from build123d import *

# Parameters (mm, degrees)
SKETCH1_W           = 80
SKETCH1_H           = 198
BOSS_EXTRUDE1_DEPTH = 5
SKETCH2_R           = 3.75
BOSS_EXTRUDE2_DEPTH = 7.5
CUT_EXTRUDE1_DEPTH  = 88.5
FILLET2_R           = 2
CUT_EXTRUDE2_START  = -5
SKETCH4_R           = 3
CUT_EXTRUDE2_DEPTH  = 2


with BuildPart() as part:
    # Sketch1 → Boss-Extrude1 (new body)
    with BuildSketch(Plane(origin=(0, 0, 0), x_dir=(1, 0, 0), z_dir=(0, 1, 0))):
        Rectangle(SKETCH1_W, SKETCH1_H)
    extrude(amount=BOSS_EXTRUDE1_DEPTH)

    # Sketch2 → Boss-Extrude2 (add)
    with BuildSketch(Plane.ZY.offset(40)):
        with Locations((-64.928905814, 3.75)):
            Circle(SKETCH2_R)
        with Locations((59.5, 3.75)):
            Circle(SKETCH2_R)
    boss_extrude2 = extrude(amount=BOSS_EXTRUDE2_DEPTH)

    # Mirror1: Boss-Extrude2 across plane
    add(boss_extrude2.mirror(Plane(origin=(0, 0, 0), x_dir=(0, 0, 1), z_dir=(1, 0, 0))))

    # Sketch3 → Cut-Extrude1 (cut, through all)
    with BuildSketch(Plane.ZY.offset(40)):
        Polygon((-99, 5), (-72.932513489, -1.759148434), (-103.799311702, -1.759148434), align=None)
    extrude(amount=-CUT_EXTRUDE1_DEPTH, mode=Mode.SUBTRACT)

    # Fillet2
    fillet2_edges = [part.edges().sort_by_distance(p)[0] for p in [
        (40, 2.5, -89.358442796),
        (-40, 2.5, -89.358442796),
    ]]
    fillet(fillet2_edges, radius=FILLET2_R)

    # Sketch4 → Cut-Extrude2 (cut)
    with BuildSketch(Plane.XZ.offset(CUT_EXTRUDE2_START)):
        with Locations((-35, -69.716885591)):
            Circle(SKETCH4_R)
        with Locations((35, -69.716885591)):
            Circle(SKETCH4_R)
        with Locations((-35, 94)):
            Circle(SKETCH4_R)
        with Locations((35, 94)):
            Circle(SKETCH4_R)
    extrude(amount=CUT_EXTRUDE2_DEPTH, mode=Mode.SUBTRACT)


solid = part.part
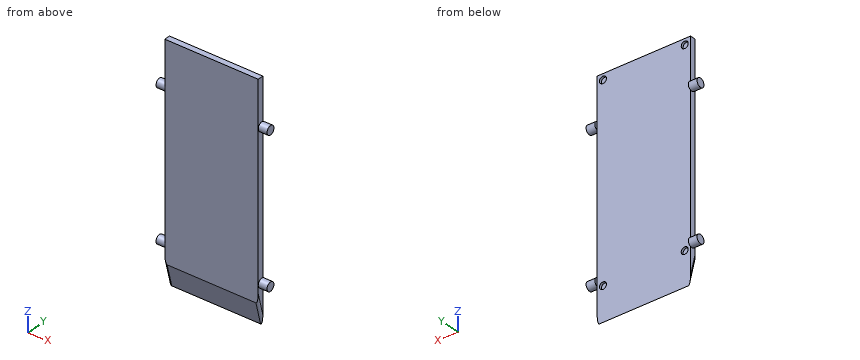
Work out the finished part from the listing and answer in its coordinate system (mm). Coordinates: 2 decimals unless noted, no trailing zeros. Write each loop counter-clockwise with the first axis right and the second up, starting at its lowest first coordinate (ties: lowest second). Pieces come first, ordered by that corner, then holes. Notation, with made-up numbers: M 26.25,0.5 L 45.25,0.5 A19 cw 45.25,27.5 Z; hole C 11.25,31 d4. An arc over 180 degrees is marked long. Answer as CSV lines item,"result". Start each with the question number.
Item 1: Flat-ended cylindrical pins translate along their axes: P1, Ø4, axis at x = 18, z = -38, coming from the +Y side; P2, Ø1.8, axis at x = 34, z = -68.5, coming from the +Y side; P3, Ø1.5, axis at y = 2.5, z = -46, coming from the +X side. Find the tip coordinate at first contact, or state that the pin passes through.
Item 2: Section B-B on x = 35 is taken. Write down the section's boundary in (y, z).
Item 3: Consider L1, parallel to Y at x = 32, z = -5; L2, parallel to Y at x = 33, z = -70; L3, parallel to X at y = 4.5, z = 77.5. Determine where each line is inside the solid, lowest interval first.
Item 4: Section C-C on z = 53 is taken. Write down the section's boundary in (x, y).
Item 5: Section A-A on z = 94 is taken. Write down the section's boundary in (x, y).
Item 6: Section D-D on x = -22 is taken. Write down the section's boundary in (y, z), and give its area (3 significant figures).
Checks:
1,P1,"stops at y = 5"
1,P2,"stops at y = 3"
1,P3,"stops at x = 40"
2,outline,"M 0,-79.72 L 5,-99 L 5,-72.72 L 3,-72.72 L 3,-66.72 L 5,-66.72 L 5,91 L 3,91 L 3,97 L 5,97 L 5,99 L 0,99 Z"
3,L1,"y = 0 to 5"
3,L2,"y = 0 to 3"
3,L3,"x = -40 to 40"
4,outline,"M -40,0 L 40,0 L 40,5 L -40,5 Z"
5,outline,"M -40,0 L 40,0 L 40,5 L 38,5 L 38,3 L 32,3 L 32,5 L -32,5 L -32,3 L -38,3 L -38,5 L -40,5 Z"
6,outline,"M 0,-79.72 L 5,-99 L 5,99 L 0,99 Z"
6,area,"942 mm²"
